Autodesk Inventor part; units mm, degrees
ref_plane "bolt_XY" through (0, 0, 0) normal (1, 0, 0) x (0, 0, -1)
ref_plane "bolt_YZ" through (0, 0, 0) normal (0, 0, -1) x (0, 1, 0)
ref_plane "bolt_ZX" through (0, 0, 0) normal (0, 1, 0) x (1, 0, 0)
sketch "Sketch_1" plane through (0, 0, 0) normal (0, 0, 1) x (1, 0, 0)
  line L0 (8, 0) -> (-5, 0)
  line L1 (-5, 0) -> (-5, 3.75)
  line L2 (-5, 3.75) -> (-4.5, 4.25)
  line L3 (-4.5, 4.25) -> (0, 4.25)
  line L4 (0, 4.25) -> (0, 2.5)
  line L5 (0, 2.5) -> (7.5095, 2.5)
  line L6 (7.5095, 2.5) -> (8, 2.0095)
  line L7 (8, 2.0095) -> (8, 0)
  line L8 (8, 0) -> (-5, 0)
revolve "Revolution1" add sketch "Sketch_1" angle 360 about axis through (8, 0, 0) along (1, 0, 0)
thread "Thread1"
sketch "Sketch2" plane through (-5, 0, 0) normal (-1, 0, 0) x (0, 0, 1)
  point P0 (0, 0)
hole "Hole1" at (-5, 0, 0) direction (1, 0, 0) diameter 4 depth 2.5 tip angle 150
sketch "Sketch_3" plane through (-5, 0, 0) normal (1, 0, 0) x (0, 0, -1)
  line L0 (-2, -1.1547) -> (0, -2.3094)
  line L1 (0, -2.3094) -> (2, -1.1547)
  line L2 (2, -1.1547) -> (2, 1.1547)
  line L3 (2, 1.1547) -> (0, 2.3094)
  line L4 (0, 2.3094) -> (-2, 1.1547)
  line L5 (-2, 1.1547) -> (-2, -1.1547)
extrude "Extrusion1" cut sketch "Sketch_3" along normal blind 2.5
ref_plane "bolt_XY" through (0, 0, 0) normal (1, 0, 0) x (0, 0, -1)
ref_plane "bolt_YZ" through (0, 0, 0) normal (0, 0, -1) x (0, 1, 0)
ref_plane "bolt_ZX" through (0, 0, 0) normal (0, 1, 0) x (1, 0, 0)
ref_plane "nut_XY" through (8, 0, 0) normal (1, 0, 0) x (0, 0, -1)
ref_plane "nut_YZ" through (8, 0, 0) normal (0, 0, -1) x (0, 1, 0)
ref_plane "nut_ZX" through (8, 0, 0) normal (0, 1, 0) x (1, 0, 0)
properties part number "SCB5-8" material "鋼"
Check sheet for the modelled part. Datum: model origin and axes. Units: mm. A direction names the side the tool comes from. Give positions to 0.01 mm unless a question says otherwise; leave off trailing zeros. Loops run counter-clockwise (first coordinate to the right, second up) from the corner with the lowest first, then second, coordinate; pieces in that order, holes last. Notation, with made-up numbers: M 14,-30 L 23,-30 A34 ccw 23,9 Z; hole C 57.25,88.5 d9. An arc over 180 degrees is marked long. Answer as CSV lines item,"result".
Item 1: Scan lines: L1, parallel to X at y = -3.25, z = 0.25; L2, parallel to Y at x = -3.75, z = -1; L3, parallel to X at y = 1.25, z = 0.25. Record each from-to range of solid material in increasing order.
Reply:
L1,"-5 to 0"
L2,"-4.13 to -1.73, 1.73 to 4.13"
L3,"-2.31 to 8"
Item 2: Set-up check for faces 1 (the face through (8, 0, 0)), 2 (the face through (-4, 0, 2)), 3 (the face through (0, 2, -2)): record each of +Z, -Z, +X, -X, +Y, -Y from which the full face is reachable in a straight line by a thin tool's end or side.
Reply:
face 1,"+Z, -Z, +X, +Y, -Y"
face 2,"-X"
face 3,"+X"
Item 3: Depth check by flat-ended pin: pin 1 Ø3 at (x, y) = (4.5, 2.5) entering from +Z; pin 2 Ø0.8 at (y, z) = (0.5, 1.5) entering from -X; pin 3 Ø1.5 at (x, z) = (4.5, -1.5) entering from -Y. Enter the tip coordinate at first touch or a pass-through.
Reply:
pin 1,"z = 2.29"
pin 2,"x = -2.49"
pin 3,"y = -2.38"
Item 4: Sectioned sample at A-A, the plane x = 6.75. Enter the section's corners in (y, z).
Reply:
outline,"C 0,0 d5"
